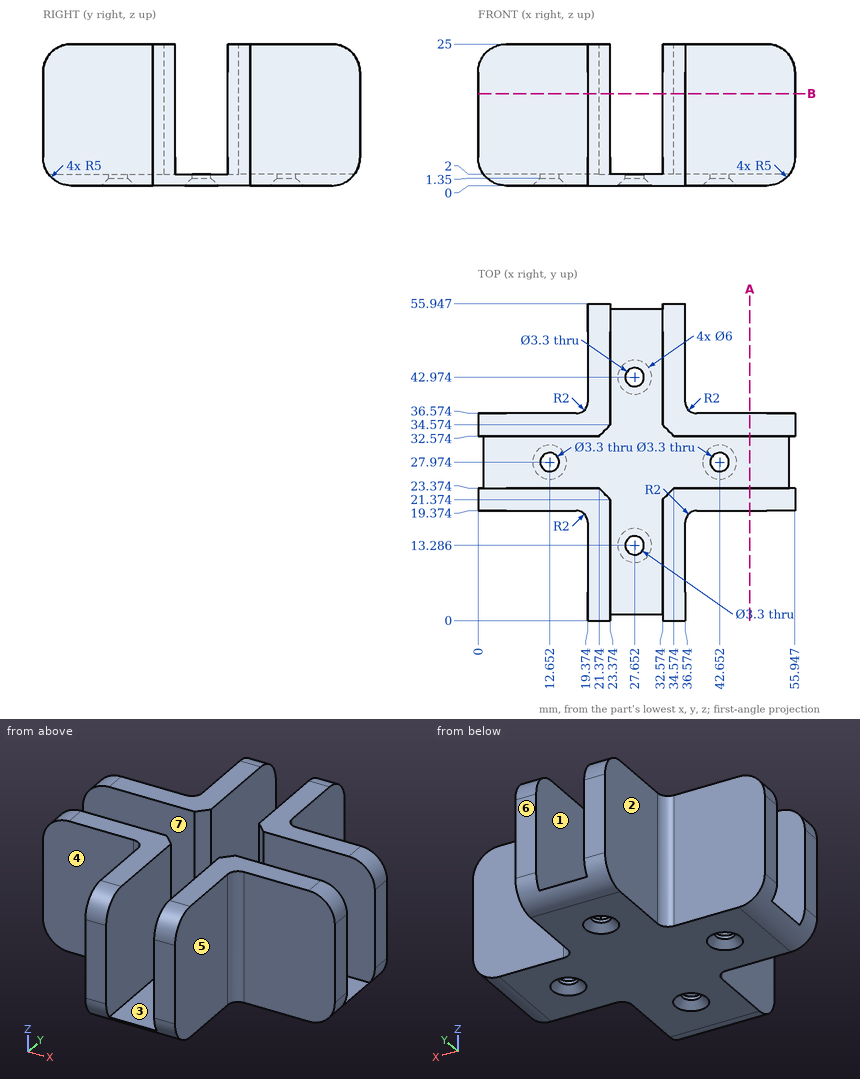
Geometry: see drawing. Coordinates: mm, zero at the bounding-box minimum. A direction names the side the tool comes from. Coordinates: 2 decimals unless noted, no trailing zeros. Loops run counter-clockwise (first coordinate to the right, second up) from the corner with the lowest first, then second, coordinate; pieces in that order, holes last. Notation, with made-up numbers: (-24, 28.25) - (24, 28.25) arc R13 cw to (24, 36.25) - close; hole circle Ø10 at (17.5, 55.25). An arc over 180 degrees is marked (long way). Put each result on its own line as item: value. Start each with the question number.
Q1. Pin query (flat end, axial travel): pin 1 Ø5 at (x, z) = (48, 10) entering from -Y; pin 2 Ø14 at (y, z) = (50, 6.5) entering from +X; pin 3 Ø6.5 at (x, z) = (13, 11) entering from +Y; pin 4 Ø1 at (x, z) = (31, 7.5) entering from -Y. Return the tip coordinate at first contact, or that it passes through.
Q2. Cut plane A-A, the plane x = 48. Return loops of the section in (y, z).
Q3. Line query: line 1 (X direction, y = 12, z = 11.25); line 2 (Y direction, x = 20, z = 17.5). Output: solid intervals per line, ascending.
Q4. Cut plane B-B, the plane z = 16.25. Give the number of separate pieces and of enclosed holes in the cut face.
Q5. Set-up query: the marked faces 1, 2 and 3. Return all of +Z, -Z, +X, -X, +Y, -Y with unobstructed straight access to the full face (end or side cutting, diameter ignored); none if empty.
Q6. Pull-direction query (Y, two-part tool) for the marked faces 4, 5, 6 and 7; classes: released by +Y, released by -Y, zero draft, split by the parting line, or undercut.
Filled sheet:
1. pin 1: y = 19.37
1. pin 2: x = 36.57
1. pin 3: y = 36.57
1. pin 4: through
2. outline: (19.37, 0) - (36.57, 0) - (36.57, 25) - (32.57, 25) - (32.57, 2) - (23.37, 2) - (23.37, 25) - (19.37, 25) - close
3. line 1: 19.37 to 23.37, 32.57 to 36.57
3. line 2: 0 to 23.37, 32.57 to 55.95
4. separate pieces: 4
4. enclosed holes: 0
5. face 1: +Z, +Y, -Y
5. face 2: +Z, -Z, -X, +Y
5. face 3: +Z
6. face 4: released by -Y
6. face 5: zero draft
6. face 6: released by +Y
6. face 7: undercut
